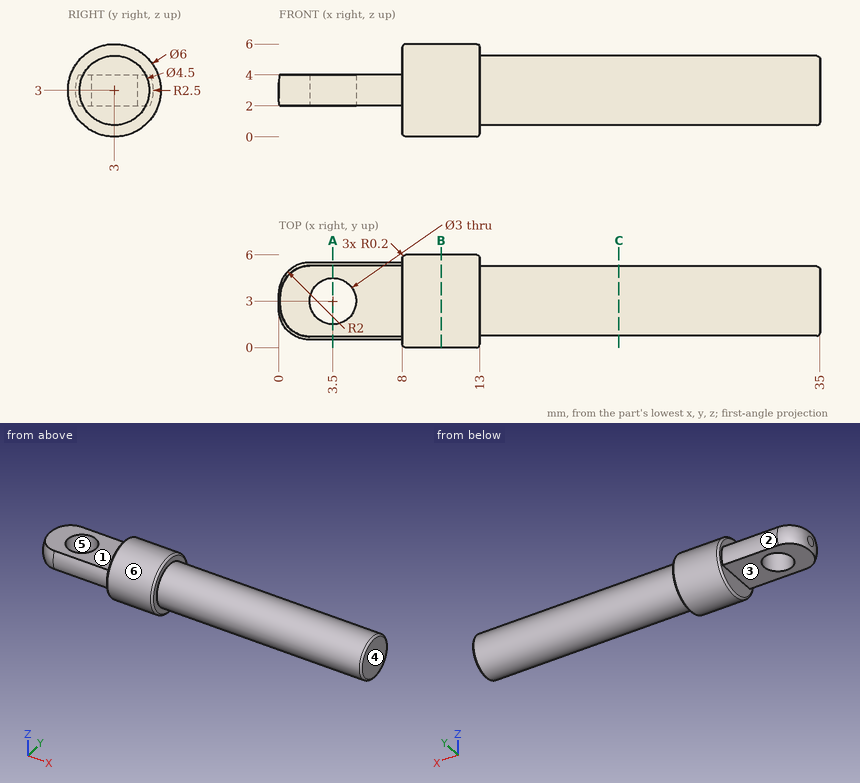
Job drawing, mm, ordinate dimensions from the low corner. One solid piece. A direction names the side the tool comes from. Round coordinates to 2 decimals unless told otherwise and drop trailing zeros. Write each loop counter-clockwise with the first axis right and the second up, starting at its lowest first coordinate (ties: lowest second). Pieces come first, ordered by that corner, then holes. Notation, with made-up numbers: M 57,-18 L 89,-18 A24 ccw 89,11 Z; hole C 59,88 d4. An arc over 180 degrees is marked long. Return JSON: item names as keys, results as strings. Group by question number.
(1) Which spindle directions (+Z, -Z, +X, -X, +Y, -Y) get a long thin tool onto all of the face, cutting with end or side? Do the marked faces 1, 2 and 3. Say none if no direction does.
(2) Saw through at A-A on x = 3.5. Write the cut outline in (y, z), then the cut area to 3 significant figures.
(3) Saw through at C-C on x = 22. Write the cut outline in (y, z), then the cut area to 3 significant figures.
(4) Drill centre lines: probe 1 along X at (y, z) = (3, 3.05); probe 2 along X at (y, z) = (0.5, 2.25); probe 3 along X at (y, z) = (2.75, 1). Where is each one in solid material? Low to high.
(5) Saw through at B-B on x = 10.5. Write the cut outline in (y, z).
(6) Two-plate mould, pull along X, no slides. Class the marked faces 4, 5 and 6: +X half, -X half, draft (parallel to the pull), parting line (faces both ways), or undercut.
(7) Pin check, flat tips, straight feed: pin 1 Ø1.5 at (x, z) = (6.5, 5) entering from +Y; pin 2 Ø2 at (x, y) = (19, 3) entering from -Z; pin 3 Ø3 at (x, z) = (5.5, 2) entering from -Y; pin 4 Ø2.5 at (x, y) = (5, 3.5) entering from -Z. Stop position of each tip, or through.
Returned:
{
 "1": {"face 1": "+Z, -X, +Y, -Y", "face 2": "-X, +Y", "face 3": "-Z, -X, +Y, -Y"},
 "2": {"outline": "M 0.71,2 L 1.5,2 L 1.5,4 L 0.71,4 A2.5 ccw Z; M 4.5,2 L 5.29,2 A2.5 ccw 5.29,4 L 4.5,4 Z", "area": "3.73 mm²"},
 "3": {"outline": "C 3,3 d4.5", "area": "15.9 mm²"},
 "4": {"probe 1": "0 to 2, 5 to 35", "probe 2": "8 to 13", "probe 3": "8 to 35"},
 "5": {"outline": "C 3,3 d6"},
 "6": {"face 4": "+X half", "face 5": "undercut", "face 6": "draft"},
 "7": {"pin 1": "through", "pin 2": "z = 0.75", "pin 3": "y = 0.5", "pin 4": "z = 2"}
}
